from build123d import *

# Parameters (mm, degrees)
SKETCH2_R          = 15
CUT_EXTRUDE1_DEPTH = 121


with BuildPart() as part:
    # Sketch1 → Revolve2 (revolve)
    with BuildSketch(Plane(origin=(0, 0, 0), x_dir=(0, 0, -1), z_dir=(1, 0, 0))):
        with BuildLine():
            Line((0, 0), (-120, 0))
            Line((-120, 0), (-120, -20))
            Line((-120, -20), (-116.242640687, -20))
            ThreePointArc((-116.242640687, -20), (-115.09459039, -19.771638598), (-114.121320344, -19.121320344))
            Line((-114.121320344, -19.121320344), (-113.757359313, -18.757359313))
            ThreePointArc((-113.757359313, -18.757359313), (-112.784089266, -18.107041059), (-111.636038969, -17.878679656))
            Line((-111.636038969, -17.878679656), (-8.363961031, -17.878679656))
            ThreePointArc((-8.363961031, -17.878679656), (-7.215910734, -18.107041059), (-6.242640687, -18.757359313))
            Line((-6.242640687, -18.757359313), (-5.878679656, -19.121320344))
            ThreePointArc((-5.878679656, -19.121320344), (-4.90540961, -19.771638598), (-3.757359313, -20))
            Line((-3.757359313, -20), (0, -20))
            Line((0, -20), (0, 0))
        make_face()
    revolve(axis=Axis((0, 0, 0), (0, 0, 1)))

    # Sketch2 → Cut-Extrude1 (cut, through all)
    with BuildSketch(Plane(origin=(0, 0, 0), x_dir=(-1, 0, 0), z_dir=(0, 0, -1))):
        Circle(SKETCH2_R)
    extrude(amount=-CUT_EXTRUDE1_DEPTH, mode=Mode.SUBTRACT)


solid = part.part
Model file for the job. Use its own axes, mm. Round coordinates to 2 decimals unless told otherwise and drop trailing zeros. Loops run counter-clockwise (first coordinate to the right, second up) from the corner with the lowest first, then second, coordinate; pieces in that order, holes last.
1. Mould opens along Z. For faces 1 (the flat face through (15, -3, 0)), 2 (the cylindrical face through (-19.524, 4.336, 1.852)), 3 (the cylindrical face through (-6.848, -16.515, 59.277)) say: +Z half, -Z half, draft (parallel to the pull), parting line (faces both ways), or undercut.
Check values:
face 1: -Z half
face 2: draft
face 3: undercut
2. Drop flat-ended pins along their axis: P1, Ø3, axis at x = 12, z = 42.5, coming from the +Y side; P2, Ø6, axis at x = 9, z = 54, coming from the -Y side; P3, Ø12, axis at x = 11, z = 22.5, coming from the -Y side; P4, Ø10, axis at x = -6, y = 1, coming from the -Z side. Give the stop position or say it passes through.
Check values:
P1: stops at y = 14.47
P2: stops at y = -16.84
P3: stops at y = -17.17
P4: passes through
3. Band-saw the part on C-C, the plane z = 97.5. List the corners of the cut face in (x, y).
Check values:
outline: circle Ø35.76 at (0, 0); hole circle Ø30 at (0, 0)
4. Wall check: probe 1 along Y at (x, z) = (-13, 99.5); probe 2 along X at (y, z) = (-4, 63); probe 3 along Z at (x, y) = (-11, 15.5). Give the ranges that are in metal, low to high.
Check values:
probe 1: y = -12.27 to -7.48, 7.48 to 12.27
probe 2: x = -17.43 to -14.46, 14.46 to 17.43
probe 3: z = 0 to 5.99, 114.01 to 120
5. Band-saw the part on A-A, the plane y = 0. List the corners of the cut face in (x, z).
Check values:
outline: (-20, 0) - (-15, 0) - (-15, 120) - (-20, 120) - (-20, 116.24) arc R3 ccw to (-19.12, 114.12) - (-18.76, 113.76) arc R3 cw to (-17.88, 111.64) - (-17.88, 8.36) arc R3 cw to (-18.76, 6.24) - (-19.12, 5.88) arc R3 ccw to (-20, 3.76) - close; (15, 0) - (20, 0) - (20, 3.76) arc R3 ccw to (19.12, 5.88) - (18.76, 6.24) arc R3 cw to (17.88, 8.36) - (17.88, 111.64) arc R3 cw to (18.76, 113.76) - (19.12, 114.12) arc R3 ccw to (20, 116.24) - (20, 120) - (15, 120) - close
